```python
from build123d import *

# Parameters (mm, degrees)
SKETCH1_R           = 15
BOSS_EXTRUDE1_DEPTH = 100
CUT_EXTRUDE1_DEPTH  = 10
SKETCH3_R           = 11
CUT_EXTRUDE2_DEPTH  = 7
SKETCH4_R           = 5
CUT_EXTRUDE3_DEPTH  = 70


with BuildPart() as part:
    # Sketch1 → Boss-Extrude1 (new body)
    with BuildSketch(Plane.XY):
        Circle(SKETCH1_R)
    extrude(amount=BOSS_EXTRUDE1_DEPTH)

    # Sketch2 → Cut-Extrude1 (cut)
    with BuildSketch(Plane.XY.offset(100)):
        with BuildLine():
            Line((-0.975, -1.029259443), (0.975, -1.029259443))
            ThreePointArc((0.975, -1.029259443), (1.339358737, -1.251570214), (1.370376634, -0.82587401))
            ThreePointArc((1.370376634, -0.82587401), (0, 1.6), (-1.370376634, -0.82587401))
            ThreePointArc((-1.370376634, -0.82587401), (-1.339358737, -1.251570214), (-0.975, -1.029259443))
        make_face()
    extrude(amount=-CUT_EXTRUDE1_DEPTH, mode=Mode.SUBTRACT)

    # Sketch3 → Cut-Extrude2 (cut)
    with BuildSketch(Plane(origin=(0, 0, 0), x_dir=(-1, 0, 0), z_dir=(0, 0, -1))):
        Circle(SKETCH3_R)
    extrude(amount=-CUT_EXTRUDE2_DEPTH, mode=Mode.SUBTRACT)

    # Sketch4 → Cut-Extrude3 (cut)
    with BuildSketch(Plane(origin=(0, 0, 7), x_dir=(-1, 0, 0), z_dir=(0, 0, -1))):
        Circle(SKETCH4_R)
    extrude(amount=-CUT_EXTRUDE3_DEPTH, mode=Mode.SUBTRACT)


solid = part.part
```
Verification items for the finished model (mm, model axes). A direction names the side the tool comes from. Round coordinates to 2 decimals unless told otherwise and drop trailing zeros. Order: outer loops, then holes, each group sorted by start corner. A loop starts at its lowest first (then second) coordinate and runs counter-clockwise, first axis right, second up. Notation, with made-up numbers: (-12.75, 62.5) -> (34.25, 62.5) arc R15 ccw to (34.25, 80.5) -> close; hole circle Ø1 at (83, 44). An arc over 180 degrees is marked (long way). Put each result on its own line as item: value. Start each with the question number.
(1) Depth check by flat-ended pin: pin 1 Ø16 at (x, y) = (0, 0) entering from -Z; pin 2 Ø4 at (x, y) = (0, 0) entering from -Z; pin 3 Ø1.5 at (y, z) = (-9.5, 47) entering from +X. Enter the tip coordinate at first touch or a pass-through.
(2) Tool access check on faces 5 (the face through (0, 0, 77)), 6 (the face through (-5, 10, 0)), 7 (the face through (0, 0, 90)). Record the directions out of +Z, -Z, +X, -X, +Y, -Y that give a thin tool (end or side, any length) a straight path to the whole face; none if there is none.
(3) Draft check along X on faces 1 (the face through (-14.985, 0.66, 49.3)), 2 (the face through (3, 0, 100)), 3 (the face through (0, 1.6, 95.1)), 4 (the face through (0, -1.029, 95)). Enter one of: +X half, -X half, draft (parallel to the pull), parting line (faces both ways), or undercut.
(4) Section check A-A (x = 0). Enter the section's corners in (y, z).
(5) Section check D-D (y = 6.75). Enter the section's corners in (x, z).
(6) Material ranges on line 1 along Y through (x, z) = (0, 34.5); line 2 along X through (y, z) = (-4.25, 57.5); line 3 along Y through (x, z) = (-1.5, 6.5), recorded low to high.
(7) Section check C-C (y = -7.5). Enter the section's corners in (x, z).
(8) Section check B-B (z = 63). Enter the section's corners in (x, y), then the cut area to 3 significant figures.
Completed:
1. pin 1: stops at z = 7
1. pin 2: stops at z = 77
1. pin 3: stops at x = 12.18
2. face 5: -Z
2. face 6: -Z, +X, -X, +Y, -Y
2. face 7: +Z
3. face 1: parting line
3. face 2: draft
3. face 3: undercut
3. face 4: undercut
4. outline: (-15, 0) -> (-11, 0) -> (-11, 7) -> (-5, 7) -> (-5, 77) -> (5, 77) -> (5, 7) -> (11, 7) -> (11, 0) -> (15, 0) -> (15, 100) -> (1.6, 100) -> (1.6, 90) -> (-1.03, 90) -> (-1.03, 100) -> (-15, 100) -> close
5. outline: (-13.4, 0) -> (-8.69, 0) -> (-8.69, 7) -> (8.69, 7) -> (8.69, 0) -> (13.4, 0) -> (13.4, 100) -> (-13.4, 100) -> close
6. line 1: y = -15 to -5, 5 to 15
6. line 2: x = -14.39 to -2.63, 2.63 to 14.39
6. line 3: y = -14.92 to -10.9, 10.9 to 14.92
7. outline: (-12.99, 0) -> (-8.05, 0) -> (-8.05, 7) -> (8.05, 7) -> (8.05, 0) -> (12.99, 0) -> (12.99, 100) -> (-12.99, 100) -> close
8. outline: circle Ø30 at (0, 0); hole circle Ø10 at (0, 0)
8. area: 628 mm2
